from build123d import *

# Parameters (mm, degrees)
SKETCH2_W                                            = 9
SKETCH2_H                                            = 9
RAIL_DEPTH                                           = 340.5
ROUNDED_EDGES_R                                      = 1
CSK_FOR_M3_FLAT_HEAD_MACHINE_SCREW1_D                = 3.4
CSK_FOR_M3_FLAT_HEAD_MACHINE_SCREW1_CSINK_D          = 6.3
CSK_FOR_M3_FLAT_HEAD_MACHINE_SCREW1_CSINK_ANGLE      = 90
CSK_FOR_M3_FLAT_HEAD_MACHINE_SCREW1_ON_F_D           = 3.4
CSK_FOR_M3_FLAT_HEAD_MACHINE_SCREW1_ON_F_CSINK_D     = 6.3
CSK_FOR_M3_FLAT_HEAD_MACHINE_SCREW1_ON_F_CSINK_ANGLE = 90


with BuildPart() as part:
    # Sketch2 → Rail (new body)
    with BuildSketch(Plane(origin=(0, 0, 0), x_dir=(1, 0, 0), z_dir=(0, 1, 0))):
        Rectangle(SKETCH2_W, SKETCH2_H)
    extrude(amount=RAIL_DEPTH)

    # Rounded Edges
    rounded_edges_edges = [part.edges().sort_by_distance(p)[0] for p in [
        (-4.5, 340.5, 0),
        (0, 340.5, 4.5),
        (4.5, 340.5, 0),
        (0, 0, 4.5),
        (-4.5, 0, 0),
        (0, 0, -4.5),
        (4.5, 0, 0),
        (0, 340.5, -4.5),
        (4.5, 170.25, 4.5),
        (-4.5, 170.25, 4.5),
        (-4.5, 170.25, -4.5),
        (4.5, 170.25, -4.5),
    ]]
    fillet(rounded_edges_edges, radius=ROUNDED_EDGES_R)

    # CSK for M3 Flat Head Machine Screw1 (through all)
    with Locations(Plane(origin=(4.5, 58.5, 0), x_dir=(0, 0, 1), z_dir=(1, 0, 0))):
        with Locations((0, 0), (0, -111.75), (0, -223.5)):
            CounterSinkHole(CSK_FOR_M3_FLAT_HEAD_MACHINE_SCREW1_D / 2, CSK_FOR_M3_FLAT_HEAD_MACHINE_SCREW1_CSINK_D / 2, counter_sink_angle=CSK_FOR_M3_FLAT_HEAD_MACHINE_SCREW1_CSINK_ANGLE)

    # CSK for M3 Flat Head Machine Screw1 on f (through all)
    with Locations(Plane(origin=(0, 307, 4.5), x_dir=(1, 0, 0), z_dir=(0, 0, 1))):
        with Locations((0, 0), (0, -91.166666667), (0, -182.333333333), (0, -273.5)):
            CounterSinkHole(CSK_FOR_M3_FLAT_HEAD_MACHINE_SCREW1_ON_F_D / 2, CSK_FOR_M3_FLAT_HEAD_MACHINE_SCREW1_ON_F_CSINK_D / 2, counter_sink_angle=CSK_FOR_M3_FLAT_HEAD_MACHINE_SCREW1_ON_F_CSINK_ANGLE)


solid = part.part
Build history of the part. All positions in model axes, mm. Round coordinates to 2 decimals unless told otherwise and drop trailing zeros. Answer as a JSON object with one key per item and string values. Group by question number.
(1) Drill centre lines: L1, parallel to Y at x = 0, z = -1.75; L2, parallel to Y at x = -0.25, z = -3; L3, parallel to Z at x = -1.75, y = 58.5. Where is each one in solid material? Low to high.
(2) Cut at A-A (z = 0). Give the number of separate pieces and of enclosed holes in the cut face, and give its area (3 significant figures).
(3) Flat gauge pins, fed straight in: pin 1 (3 mm diameter, centred on x = 0, y = 124.67, fed in from -Z); pin 2 (4 mm diameter, centred on y = 282, z = 0, fed in from +X). Where does each tip first touch, or does it go through?
Responses:
{
 "1": {"L1": "y = 0 to 31.8, 35.2 to 122.97, 126.37 to 214.13, 217.53 to 305.3, 308.7 to 340.5", "L2": "y = 0 to 31.82, 35.18 to 122.99, 126.35 to 214.15, 217.51 to 305.32, 308.68 to 340.5", "L3": "z = -4.5 to -1.7, 1.7 to 4.5"},
 "2": {"separate pieces": "4", "enclosed holes": "4", "area": "2,930 mm2"},
 "3": {"pin 1": "passes through", "pin 2": "stops at x = 3.35"}
}
